from build123d import *

# Parameters (mm, degrees)
EXTRUDE_1_DEPTH      = 50
SHELL_1_T            = -5
EXTRUDE_2_DEPTH      = 5
SKETCH_10_R          = 2.35
EXTRUDE_3_DEPTH      = 5
CUT_EXTRUDE_1_DEPTH  = 5
EXTRUDE_START        = -30
EXTRUDE_4_DEPTH      = 30
SHELL_START          = -13
SHELL_13_DEPTH       = 8
SHELL_START_2        = -43
SHELL_13_2_DEPTH     = 30
SHELL_13_3_OUTLINE_R = 4.35
SHELL_13_3_DEPTH     = 1
SHELL_START_3        = -8
SHELL_13_4_DEPTH     = 3
SHELL_START_4        = -5
SHELL_13_5_DEPTH     = 3
SHELL_13_6_DEPTH     = 26
CUT_EXTRUDE_2_DEPTH  = 144.120865122
CUT_EXTRUDE_3_DEPTH  = 5


# Read off the part's stored shape, not the designer's step: 凸台-拉伸4, 抽壳13
with BuildPart() as part:
    # 草图3 → 凸台-拉伸1 (new body)
    with BuildSketch(Plane(origin=(0, 0, 0), x_dir=(1, 0, 0), z_dir=(0, 1, 0))):
        Polygon((57.849497127, -89.790549593), (-101.961949946, -31.82244298), (-57.849497127, 89.790549593), (101.961949946, 31.82244298), align=None)
    extrude(amount=-EXTRUDE_1_DEPTH)

    # 抽壳1
    shell_1_openings = [part.faces().sort_by_distance(p)[0] for p in [
        (0, 0, 0),
    ]]
    offset(amount=SHELL_1_T, openings=shell_1_openings, kind=Kind.INTERSECTION)

    # 草图4 → 凸台-拉伸2 (add)
    with BuildSketch(Plane(origin=(0, -10, 0), x_dir=(1, 0, 0), z_dir=(0, 1, 0))):
        Polygon((-54.85410476, 83.385268602), (95.556668956, 28.827050613), (54.793783145, -83.551568403), (-95.616990571, -28.993350414), align=None)
        with BuildLine():
            Line((-33.405753886, 43.6927409), (-49.102625926, 49.386437869))
            ThreePointArc((-49.102625926, 49.386437869), (-50.631828553, 49.317990247), (-51.664738322, 48.188280923))
            Line((-51.664738322, 48.188280923), (-70.544015322, -3.859728807))
            ThreePointArc((-70.544015322, -3.859728807), (-70.4755677, -5.388931433), (-69.345858375, -6.421841203))
            Line((-69.345858375, -6.421841203), (-53.648986335, -12.115538173))
            ThreePointArc((-53.648986335, -12.115538173), (-18.754387434, -51.703703465), (33.405753886, -43.6927409))
            Line((33.405753886, -43.6927409), (49.102625926, -49.386437869))
            ThreePointArc((49.102625926, -49.386437869), (50.631828553, -49.317990247), (51.664738322, -48.188280923))
            Line((51.664738322, -48.188280923), (70.544015322, 3.859728807))
            ThreePointArc((70.544015322, 3.859728807), (70.4755677, 5.388931433), (69.345858375, 6.421841203))
            Line((69.345858375, 6.421841203), (53.648986335, 12.115538173))
            ThreePointArc((53.648986335, 12.115538173), (18.754387434, 51.703703465), (-33.405753886, 43.6927409))
        make_face(mode=Mode.SUBTRACT)
    extrude(amount=EXTRUDE_2_DEPTH)

    # 草图10 → 凸台-拉伸3 (add)
    with BuildSketch(Plane(origin=(0, -10, 0), x_dir=(1, 0, 0), z_dir=(0, 1, 0))):
        Polygon((-54.85410476, 83.385268602), (95.556668956, 28.827050613), (54.87017905, -83.340953621), (-95.540594666, -28.782735632), align=None)
        with Locations(Location((44.109349089, -16.22853422, 0), (0, 0, 270))):
            Circle(SKETCH_10_R, mode=Mode.SUBTRACT)
        with Locations(Location((-44.109349089, 16.22853422, 0), (0, 0, 270))):
            Circle(SKETCH_10_R, mode=Mode.SUBTRACT)
        Polygon((5.990784733, -12.810561982), (-31.611908696, 0.828992516), (-24.792131447, 19.63033923), (12.810561982, 5.990784733), align=None, mode=Mode.SUBTRACT)
    extrude(amount=-EXTRUDE_3_DEPTH)

    # 草图11 → 切除-拉伸1 (cut)
    with BuildSketch(Plane(origin=(0, -45, 0), x_dir=(1, 0, 0), z_dir=(0, 1, 0))):
        Polygon((57.849497127, -89.790549593), (101.961949946, 31.82244298), (-57.849497127, 89.790549593), (-101.961949946, -31.82244298), align=None)
    extrude(amount=-CUT_EXTRUDE_1_DEPTH, mode=Mode.SUBTRACT)

    # 凸台-拉伸4 outline → 凸台-拉伸4 (add)
    # profile 1 of 4: a face of its own
    with BuildSketch(Plane.XZ.offset(45).offset(EXTRUDE_START)):
        Polygon((92.146780331, -19.426377256), (82.746106974, -22.83626588), (86.155995598, -32.236939238), (95.556668956, -28.827050613), align=None)
        Polygon((91.713500361, -27.029815193), (87.953231018, -28.393770643), (86.589275569, -24.6335013), (90.349544911, -23.26954585), align=None, mode=Mode.SUBTRACT)
    # profile 2 of 4: a face of its own
    with BuildSketch(Plane.XZ.offset(45).offset(EXTRUDE_START)):
        Polygon((-54.85410476, -83.385268602), (-45.453403196, -79.975369746), (-48.863293462, -70.574691864), (-58.263966819, -73.984580488), align=None)
        Polygon((-49.296573432, -78.178129801), (-53.056842775, -79.542085251), (-54.420798224, -75.781815908), (-50.660528881, -74.417860458), align=None, mode=Mode.SUBTRACT)
    # profile 3 of 4: a face of its own
    with BuildSketch(Plane.XZ.offset(45).offset(EXTRUDE_START)):
        Polygon((49.11739228, 70.666865773), (58.263993385, 73.984595245), (54.87017905, 83.340953621), (54.85410476, 83.385268602), (45.453431403, 79.975379978), align=None)
        Polygon((50.660555447, 74.417875215), (49.296599998, 78.178144558), (53.05686934, 79.542100008), (54.42082479, 75.781830665), align=None, mode=Mode.SUBTRACT)
    # profile 4 of 4: a face of its own
    with BuildSketch(Plane.XZ.offset(45).offset(EXTRUDE_START)):
        Polygon((-95.540594666, 28.782735632), (-92.146780332, 19.426377256), (-82.746106974, 22.83626588), (-86.155995598, 32.236939238), (-95.556668956, 28.827050613), align=None)
        Polygon((-91.713500361, 27.029815193), (-87.953231018, 28.393770643), (-86.589275569, 24.6335013), (-90.349544911, 23.26954585), align=None, mode=Mode.SUBTRACT)
    extrude(amount=EXTRUDE_4_DEPTH)

    # 抽壳13 outline → 抽壳13 (cut)
    with BuildSketch(Plane(origin=(0, 0, 0), x_dir=(1, 0, 0), z_dir=(0, 1, 0)).offset(SHELL_START)):
        Polygon((-99.39983755, -30.624286033), (56.65134018, -87.228437197), (99.39983755, 30.624286033), (-56.65134018, 87.228437197), align=None)
        Polygon((57.432291447, -82.142796675), (56.052261707, -85.947380999), (-98.118781352, -30.02520756), (-96.738751612, -26.220623236), align=None, mode=Mode.SUBTRACT)
        with BuildLine():
            Line((-72.424149993, -3.177751082), (-53.544872994, 48.870258648))
            ThreePointArc((-53.544872994, 48.870258648), (-51.479053454, 51.129677297), (-48.420648201, 51.266572541))
            Line((-48.420648201, 51.266572541), (-33.739920947, 45.941459864))
            ThreePointArc((-33.739920947, 45.941459864), (19.436365158, 53.583838136), (55.347108846, 13.627088551))
            Line((55.347108846, 13.627088551), (70.0278361, 8.301975874))
            ThreePointArc((70.0278361, 8.301975874), (72.28725475, 6.236156335), (72.424149993, 3.177751082))
            Line((72.424149993, 3.177751082), (53.544872994, -48.870258648))
            ThreePointArc((53.544872994, -48.870258648), (51.479053454, -51.129677297), (48.420648201, -51.266572541))
            Line((48.420648201, -51.266572541), (33.739920947, -45.941459864))
            ThreePointArc((33.739920947, -45.941459864), (-19.436365158, -53.583838136), (-55.347108846, -13.627088551))
            Line((-55.347108846, -13.627088551), (-70.0278361, -8.301975874))
            ThreePointArc((-70.0278361, -8.301975874), (-72.28725475, -6.236156335), (-72.424149993, -3.177751082))
        make_face(mode=Mode.SUBTRACT)
    extrude(amount=SHELL_13_DEPTH, mode=Mode.SUBTRACT)

    # Shell 13 2 outline → Shell 13 2 (cut)
    with BuildSketch(Plane(origin=(0, 0, 0), x_dir=(1, 0, 0), z_dir=(0, 1, 0)).offset(SHELL_START_2)):
        Polygon((-99.39983755, -30.624286033), (56.65134018, -87.228437197), (99.39983755, 30.624286033), (-56.65134018, 87.228437197), align=None)
        Polygon((56.641948324, -75.523741054), (54.612089439, -81.119830088), (57.432291447, -82.142796675), (56.052261707, -85.947380999), (-98.118781352, -30.02520756), (-96.738751612, -26.220623236), (-93.918549605, -27.243589823), (-91.88869072, -21.64750079), (-94.708892728, -20.624534203), (-56.052261707, 85.947380999), (-52.291964157, 84.583415318), (-53.314932385, 81.763208785), (-47.674528371, 79.71727561), (-46.651560142, 82.537482143), (88.718107995, 33.435096184), (87.695141407, 30.614894177), (94.275612757, 28.22797214), (91.88869072, 21.64750079), (94.708892728, 20.624534203), (59.462150331, -76.546707641), align=None, mode=Mode.SUBTRACT)
    extrude(amount=SHELL_13_2_DEPTH, mode=Mode.SUBTRACT)

    # Shell 13 3 outline → Shell 13 3 (cut)
    with BuildSketch(Plane(origin=(0, 0, 0), x_dir=(1, 0, 0), z_dir=(0, 1, 0)).offset(SHELL_START)):
        with BuildLine():
            ThreePointArc((-48.420648201, 51.266572541), (-51.479053454, 51.129677297), (-53.544872994, 48.870258648))
            Line((-53.544872994, 48.870258648), (-72.424149993, -3.177751082))
            ThreePointArc((-72.424149993, -3.177751082), (-72.28725475, -6.236156335), (-70.0278361, -8.301975874))
            Line((-70.0278361, -8.301975874), (-55.347108846, -13.627088551))
            ThreePointArc((-55.347108846, -13.627088551), (-19.436365158, -53.583838136), (33.739920947, -45.941459864))
            Line((33.739920947, -45.941459864), (48.420648201, -51.266572541))
            ThreePointArc((48.420648201, -51.266572541), (51.479053454, -51.129677297), (53.544872994, -48.870258648))
            Line((53.544872994, -48.870258648), (72.424149993, 3.177751082))
            ThreePointArc((72.424149993, 3.177751082), (72.28725475, 6.236156335), (70.0278361, 8.301975874))
            Line((70.0278361, 8.301975874), (55.347108846, 13.627088551))
            ThreePointArc((55.347108846, 13.627088551), (19.436365158, 53.583838136), (-33.739920947, 45.941459864))
            Line((-33.739920947, 45.941459864), (-48.420648201, 51.266572541))
        make_face()
        with Locations((44.109349089, -16.22853422)):
            Circle(SHELL_13_3_OUTLINE_R, mode=Mode.SUBTRACT)
        with Locations((-44.109349089, 16.22853422)):
            Circle(SHELL_13_3_OUTLINE_R, mode=Mode.SUBTRACT)
        Polygon((15.372674378, 7.18894168), (7.18894168, -15.372674378), (-34.174021092, -0.369164431), (-25.990288394, 22.192451627), align=None, mode=Mode.SUBTRACT)
    extrude(amount=SHELL_13_3_DEPTH, mode=Mode.SUBTRACT)

    # Shell 13 4 outline → Shell 13 4 (cut)
    with BuildSketch(Plane(origin=(0, 0, 0), x_dir=(1, 0, 0), z_dir=(0, 1, 0)).offset(SHELL_START_3)):
        Polygon((56.052261707, -85.947380999), (57.432291447, -82.142796675), (-96.738751612, -26.220623236), (-98.118781352, -30.02520756), align=None)
    extrude(amount=SHELL_13_4_DEPTH, mode=Mode.SUBTRACT)

    # Shell 13 5 outline → Shell 13 5 (cut)
    with BuildSketch(Plane(origin=(0, 0, 0), x_dir=(1, 0, 0), z_dir=(0, 1, 0)).offset(SHELL_START_4)):
        Polygon((-99.39983755, -30.624286033), (56.65134018, -87.228437197), (99.39983755, 30.624286033), (-56.65134018, 87.228437197), align=None)
        Polygon((59.462150331, -76.546707641), (56.052261707, -85.947380999), (-98.118781352, -30.02520756), (-94.708892728, -20.624534203), (-56.052261707, 85.947380999), (-46.651560142, 82.537482143), (88.718107995, 33.435096184), (98.118781352, 30.02520756), (94.708892728, 20.624534203), align=None, mode=Mode.SUBTRACT)
    extrude(amount=SHELL_13_5_DEPTH, mode=Mode.SUBTRACT)

    # Shell 13 6 outline → Shell 13 6 (cut)
    with BuildSketch(Plane(origin=(0, 0, 0), x_dir=(1, 0, 0), z_dir=(0, 1, 0)).offset(SHELL_START_2)):
        Polygon((54.612089439, -81.119830088), (54.255026287, -82.104212404), (47.700648719, -79.726755316), (46.601460456, -82.519309577), (56.052261707, -85.947380999), (57.432291447, -82.142796675), align=None)
        Polygon((-94.275612757, -28.22797214), (-93.918549605, -27.243589823), (-96.738751612, -26.220623236), (-98.118781352, -30.02520756), (-88.718107995, -33.435096184), (-87.695141407, -30.614894177), align=None)
    extrude(amount=SHELL_13_6_DEPTH, mode=Mode.SUBTRACT)

    # 草图16 → 切除-拉伸2 (cut, through all)
    with BuildSketch(Plane.XZ.offset(45)):
        Polygon((-101.961949946, 31.82244298), (57.849497127, 89.790549593), (101.961949946, -31.82244298), (-57.849497127, -89.790549593), align=None)
        Polygon((-100.680893748, 31.223364506), (-57.250418654, -88.509493395), (100.680893748, -31.223364506), (57.250418654, 88.509493395), align=None, mode=Mode.SUBTRACT)
    extrude(amount=-CUT_EXTRUDE_2_DEPTH, mode=Mode.SUBTRACT)

    # 草图17 → 切除-拉伸3 (cut)
    with BuildSketch(Plane(origin=(0, 0, 0), x_dir=(1, 0, 0), z_dir=(0, 1, 0))):
        Polygon((57.250418654, -88.509493395), (-100.680893748, -31.223364506), (-57.250418654, 88.509493395), (100.680893748, 31.223364506), align=None)
    extrude(amount=-CUT_EXTRUDE_3_DEPTH, mode=Mode.SUBTRACT)


solid = part.part
CAD build for the part. Positions are in the model's coordinates, mm. A direction names the side the tool comes from. Give positions to 0.01 mm unless a question says otherwise; leave off trailing zeros. Order: outer loops, then holes, each group sorted by start corner. A loop starts at its lowest first (then second) coordinate and runs counter-clockwise, first axis right, second up. Notation, with made-up numbers: (66.25, -22) -> (100.25, -22) arc R36 cw to (100.25, 14) -> close; hole circle Ø10 at (-13, 32.5). An arc over 180 degrees is marked (long way). Return JSON: item names as keys, results as strings.
Q1. Saw through at C-C (y = -33). Count the separate pieces of the cut face and the enclosed holes in it, then the cut area to 3 significant figures.
Working result:
{"separate pieces": "2", "enclosed holes": "6", "area": "1,880 mm²"}
Q2. Saw through at B-B (x = 22). Write the cut outline in (y, z), then the cut area to 3 significant figures.
Working result:
{"outline": "(-45, -59.76) -> (-5, -59.76) -> (-5, -58.7) -> (-43, -58.7) -> (-43, -57.64) -> (-13, -57.64) -> (-13, 69.29) -> (-8, 69.29) -> (-8, 73.6) -> (-43, 73.6) -> (-43, 74.66) -> (-5, 74.66) -> (-5, 75.72) -> (-45, 75.72) -> (-45, 71.47) -> (-10, 71.47) -> (-10, 71.42) -> (-15, 71.42) -> (-15, -55.51) -> (-45, -55.51) -> close; (-12, -52.58) -> (-5, -52.58) -> (-5, -50.41) -> (-10, -50.41) -> (-10, 50.41) -> (-5, 50.41) -> (-5, 52.58) -> (-12, 52.58) -> close", "area": "733 mm²"}
Q3. Mould opens along X. For faces 4 (the face through (20.09, -28.21, -58.33)), 5 (the face through (20.61, -25.28, -60.267)), 6 (the face through (-79.27, -25.28, -27.8)) say: pulls with the +X half, pulls with the -X half, needs draft (parallel to the pull), parting line crosses it, or undercut.
Working result:
{"face 4": "undercut", "face 5": "pulls with the +X half", "face 6": "pulls with the -X half"}
Q4. Drill centre lines: line 1 (Z direction, x = -45, y = -21); line 2 (Z direction, x = 52, y = -15.5); line 3 (Z direction, x = -19.5, y = -35). Where is each one in solid material? Low to high.
Working result:
{"line 1": "-84.07 to -83, -81.94 to -79.81, 47.17 to 49.29, 50.36 to 51.42", "line 2": "-48.88 to -47.82, -46.75 to -44.63, 71.71 to 74.9, 79.16 to 84.48, 85.54 to 86.61", "line 3": "-74.82 to -73.75, -72.69 to -70.56, 56.41 to 58.54, 59.61 to 60.67"}
Q5. Saw through at A-A (z = 40). Write the cut outline in (x, y).
Working result:
{"outline": "(-76.48, -45) -> (-64.75, -45) -> (-64.75, -10) -> (-64.62, -10) -> (-64.62, -15) -> (70.59, -15) -> (70.59, -45) -> (74.85, -45) -> (74.85, -5) -> (73.78, -5) -> (73.78, -43) -> (72.72, -43) -> (72.72, -13) -> (-58.75, -13) -> (-58.75, -8) -> (-70.62, -8) -> (-70.62, -43) -> (-73.55, -43) -> (-73.55, -5) -> (-76.48, -5) -> close; (-40.61, -12) -> (56.76, -12) -> (56.76, -5) -> (54.63, -5) -> (54.63, -10) -> (-37.75, -10) -> (-37.75, -5) -> (-40.61, -5) -> close"}
Q6. Saw through at D-D (x = 80). Write the cut outline in (y, z), then the cut area to 3 significant figures.
Working result:
{"outline": "(-45, -38.72) -> (-5, -38.72) -> (-5, -37.66) -> (-43, -37.66) -> (-43, -36.6) -> (-13, -36.6) -> (-13, 19.93) -> (-43, 19.93) -> (-43, 22.86) -> (-5, 22.86) -> (-5, 25.79) -> (-45, 25.79) -> (-45, 14.06) -> (-15, 14.06) -> (-15, -34.47) -> (-45, -34.47) -> close", "area": "521 mm²"}
Q7. Flat gauge pins, fed straight in: pin 1 (2.5 mm diameter, centred on x = -88.5, z = 25.5, fed in from -Y); pin 2 (3 mm diameter, centred on y = -16.5, z = -24.5, fed in from +X); pin 3 (5.5 mm diameter, centred on x = -44.11, z = -16.23, fed in from +Y). Where does each tip first touch, or does it go through?
Working result:
{"pin 1": "y = -15", "pin 2": "x = 98.79", "pin 3": "y = -10"}
Q8. Which spindle directions (+Z, -Z, +X, -X, +Y, -Y) get a long thin tool onto all of the face, cutting with end or side? Do faces 1 (the face through (72.268, -8.549, -6.276)), 2 (the face through (-39.96, -12.51, -17.54)), 3 (the face through (-52, -15, -77)). Say none if no direction does.
Working result:
{"face 1": "+Y", "face 2": "none", "face 3": "-Y"}
